from build123d import *

# Parameters (mm, degrees)
EXTRUDE_1_DEPTH             = 10
HOLE_WIZARD_M31_D           = 2.5
HOLE_WIZARD_M31_CSINK_D     = 3.2
HOLE_WIZARD_M31_CSINK_ANGLE = 110
HOLE_WIZARD_M32_D           = 2.5
HOLE_WIZARD_M32_CSINK_D     = 3.3
HOLE_WIZARD_M32_CSINK_ANGLE = 110


with BuildPart() as part:
    # Эскиз1 → Бобышка-Вытянуть1 (new body)
    with BuildSketch(Plane.XY):
        Polygon((0, 0), (0, 18), (2.309401077, 18), (10, 4.679491924), (10, 0), align=None)
    extrude(amount=EXTRUDE_1_DEPTH)

    # Отверстие обработанное метчиком M31 (through all)
    with Locations(Plane.ZY):
        with Locations((5, 13)):
            CounterSinkHole(HOLE_WIZARD_M31_D / 2, HOLE_WIZARD_M31_CSINK_D / 2, counter_sink_angle=HOLE_WIZARD_M31_CSINK_ANGLE)

    # Отверстие обработанное метчиком M32 (through all)
    with Locations(Plane.XZ):
        with Locations((7, 5)):
            CounterSinkHole(HOLE_WIZARD_M32_D / 2, HOLE_WIZARD_M32_CSINK_D / 2, counter_sink_angle=HOLE_WIZARD_M32_CSINK_ANGLE)


solid = part.part
Source: CAD feature listing. Evaluate the final solid. Frame: model axes, mm. Round coordinates to 2 decimals unless told otherwise and drop trailing zeros. Write each loop counter-clockwise with the first axis right and the second up, starting at its lowest first coordinate (ties: lowest second). Pieces come first, ordered by that corner, then holes. Notation, with made-up numbers: (52, 0.5) - (78, 0.5) arc R26 ccw to (78, 36.5) - close; hole circle Ø7 at (75, 35). An arc over 180 degrees is marked (long way). Use CSV: the item, a comma, the result in double quotes. Start each with the question number.
(1) Material intervals for probe 1 along X at (y, z) = (3, 5); probe 2 along Z at (x, y) = (3.35, 13); probe 3 along Y at (x, z) = (3, 5), sorted ascending. Write a range as [from, to].
(2) Cut plane B-B, the plane z = 2. Return loops of the section in (x, y).
(3) Cut plane A-A, the plane y = 1.75. Return loops of the section in (x, z), and give its area (3 significant figures).
(4) First-contact query: pin 1 Ø3 at (y, z) = (13, 5) entering from +X; pin 2 Ø2 at (x, z) = (7, 5) entering from -Y; pin 3 Ø4 at (x, z) = (7, 8) entering from +Y. Flat tips, straight axial feed; report the tip coordinate or a pass-through.
(5) Cut plane D-D, the plane y = 13. Return loops of the section in (x, z), and give its area (3 significant figures).
(6) Cut plane C-C, the plane x = 7. Return loops of the section in (y, z).
(7) Mould query, pull axis X, two halves, no side actions, for faces 1 (the face through (4, 7, 10)), 2 (the face through (10, 2, 5)), 3 (the face through (5.845, 4.863, 4.521)). Classes: pulls with the +X half, pulls with the -X half, needs draft (parallel to the pull), parting line crosses it, or undercut.
Geometry says:
1,probe 1,"[0, 5.75], [8.25, 10]"
1,probe 2,"[0, 3.75], [6.25, 10]"
1,probe 3,"[0, 11.75], [14.25, 16.8]"
2,outline,"(0, 0) - (10, 0) - (10, 4.68) - (2.31, 18) - (0, 18) - close"
3,outline,"(0, 0) - (10, 0) - (10, 10) - (0, 10) - close; hole circle Ø2.5 at (7, 5)"
3,area,"95.1 mm²"
4,pin 1,"x = 5.96"
4,pin 2,"through"
4,pin 3,"y = 13.34"
5,outline,"(0, 0) - (5.2, 0) - (5.2, 3.75) - (0.25, 3.75) - (0, 3.4) - close; (0, 6.6) - (0.25, 6.25) - (5.2, 6.25) - (5.2, 10) - (0, 10) - close"
5,area,"38.9 mm²"
6,outline,"(0, 0) - (9.88, 0) - (9.88, 3.75) - (0.28, 3.75) - (0, 3.35) - close; (0, 6.65) - (0.28, 6.25) - (9.88, 6.25) - (9.88, 10) - (0, 10) - close"
7,face 1,"needs draft"
7,face 2,"pulls with the +X half"
7,face 3,"undercut"
